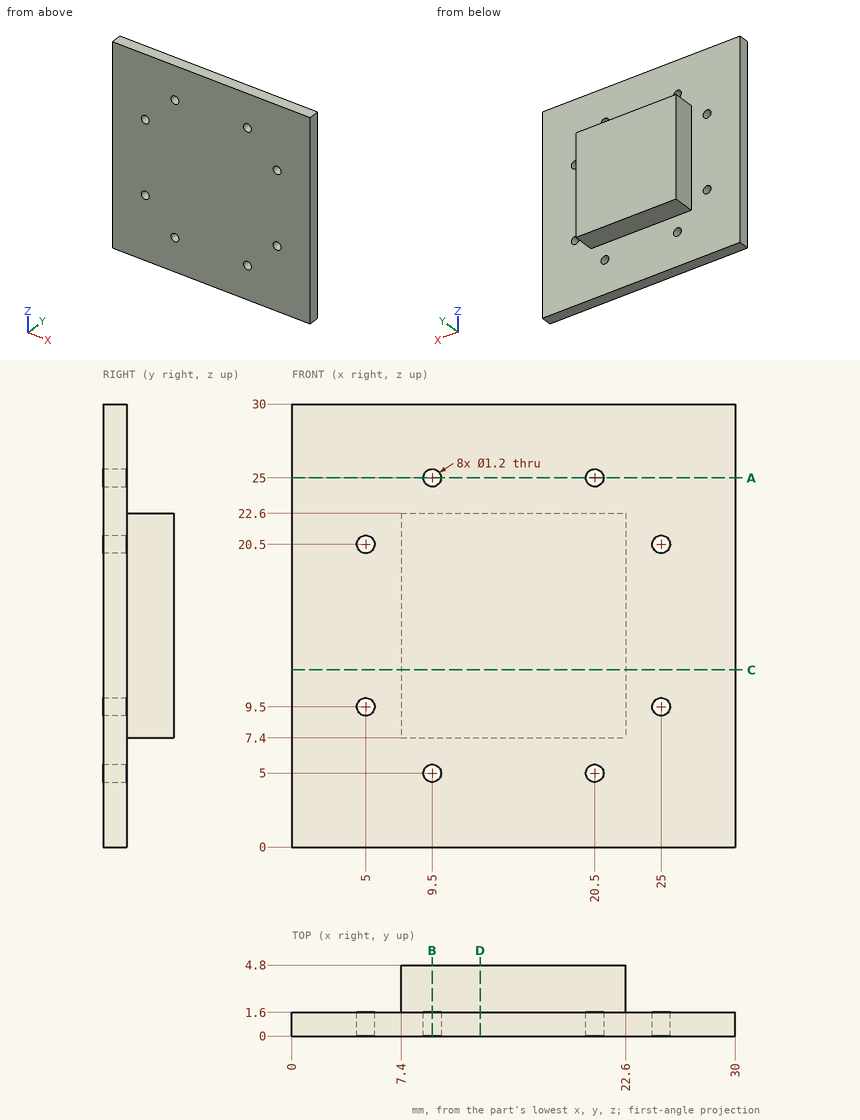
Verification items for this drawing (mm, ordinates from the low corner). Round coordinates to 2 decimals unless told otherwise and drop trailing zeros. Order: outer loops, then holes, each group sorted by start corner. A loop starts at its lowest first (then second) coordinate and runs counter-clockwise, first axis right, second up. Notation, with made-up numbers: M 10,59.25 L 48,59.25 A17 cw 48,75.25 Z; hole C 81.25,75 d4. An arc over 180 degrees is marked long. Answer in a Markdown table with one row per item. Add a question column.
Item 1: Sectioned sample at C-C, the plane z = 12. Enter the section's corners in (x, y).
Item 2: Sectioned sample at B-B, the plane x = 9.5. Enter the section's corners in (y, z), plus the area to 3 significant figures.
Item 3: Depth check by flat-ended pin: pin 1 Ø2.5 at (y, z) = (3, 17.5) entering from -X; pin 2 Ø1.4 at (x, z) = (20.5, 5) entering from +Y; pin 3 Ø1.6 at (x, y) = (17, 4) entering from -Z. Enter the tip coordinate at first touch or a pass-through.
Item 4: Material ranges on L1, parallel to X at y = 0.6, z = 5; L2, parallel to X at y = 0.9, z = 20.5, recorded low to high. Write a range as [from, to].
Item 5: Sectioned sample at A-A, the plane z = 25. Enter the section's corners in (x, y).
Item 6: Sectioned sample at D-D, the plane x = 12.75. Enter the section's corners in (y, z).
Filled in:
| question | item | result |
|---|---|---|
| 1 | outline | M 0,0 L 30,0 L 30,1.6 L 22.6,1.6 L 22.6,4.8 L 7.4,4.8 L 7.4,1.6 L 0,1.6 Z |
| 2 | outline | M 0,0 L 1.6,0 L 1.6,4.4 L 0,4.4 Z; M 0,5.6 L 1.6,5.6 L 1.6,7.4 L 4.8,7.4 L 4.8,22.6 L 1.6,22.6 L 1.6,24.4 L 0,24.4 Z; M 0,25.6 L 1.6,25.6 L 1.6,30 L 0,30 Z |
| 2 | area | 92.8 mm² |
| 3 | pin 1 | stops at x = 7.4 |
| 3 | pin 2 | stops at y = 1.6 |
| 3 | pin 3 | stops at z = 7.4 |
| 4 | L1 | x = [0, 8.9], [10.1, 19.9], [21.1, 30] |
| 4 | L2 | x = [0, 4.4], [5.6, 24.4], [25.6, 30] |
| 5 | outline | M 0,0 L 8.9,0 L 8.9,1.6 L 0,1.6 Z; M 10.1,0 L 19.9,0 L 19.9,1.6 L 10.1,1.6 Z; M 21.1,0 L 30,0 L 30,1.6 L 21.1,1.6 Z |
| 6 | outline | M 0,0 L 1.6,0 L 1.6,7.4 L 4.8,7.4 L 4.8,22.6 L 1.6,22.6 L 1.6,30 L 0,30 Z |
